Work out the finished part from the listing and answer in its coordinate system (mm). Face numbers are marked on the shaded views. Coordinates: 2 decimals unless noted, no trailing zeros. Order: outer loops, then holes, each group sorted by start corner. A loop starts at its lowest first (then second) coordinate and runs counter-clockwise, first axis right, second up. Notation, with made-up numbers: M 82,54.25 L 138,54.25 A27 ccw 138,73.25 Z; hole C 86.5,-3.5 d7. An arc over 180 degrees is marked long. Use a Markdown table: item, result.
from build123d import *

# Parameters (mm, degrees)
BOSS_EXTRUDE1_DEPTH = 55
SKETCH2_R           = 1.5
CUT_EXTRUDE1_DEPTH  = 10


with BuildPart() as part:
    # Sketch1 → Boss-Extrude1 (new body)
    with BuildSketch(Plane(origin=(0, 0, 0), x_dir=(1, 0, 0), z_dir=(0, 1, 0))):
        Polygon((3.175426481, 0), (1.58771324, 2.75), (-1.58771324, 2.75), (-3.175426481, 0), (-1.58771324, -2.75), (1.58771324, -2.75), align=None)
    extrude(amount=BOSS_EXTRUDE1_DEPTH)

    # Sketch2 → Cut-Extrude1 (cut)
    with BuildSketch(Plane(origin=(0, 55, 0), x_dir=(1, 0, 0), z_dir=(0, 1, 0))):
        with Locations(Location((0, 0, 0), (0, 0, 270))):
            Circle(SKETCH2_R)
    cut_extrude1 = extrude(amount=-CUT_EXTRUDE1_DEPTH, mode=Mode.SUBTRACT)

    # Mirror1: Cut-Extrude1 across plane
    add(cut_extrude1.mirror(Plane(origin=(0, 27.5, 0), x_dir=(0, 0, 1), z_dir=(0, -1, 0))), mode=Mode.SUBTRACT)


solid = part.part
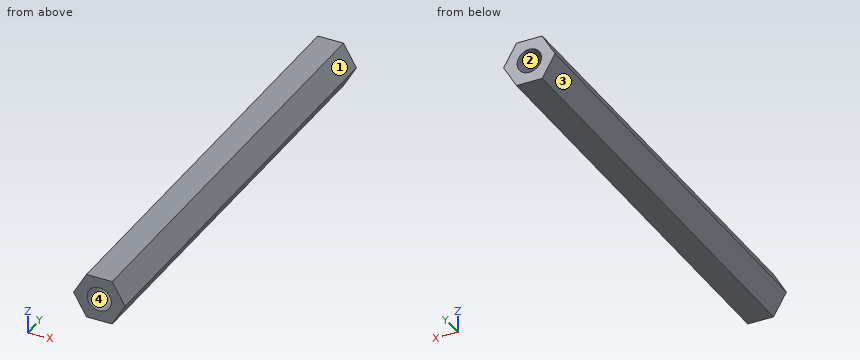
1. Section B-B on x = 0 is taken. Determine the outline of the cut face in (y, z).
Answers below:
| item | result |
|---|---|
| outline | M 0,-2.75 L 55,-2.75 L 55,-1.5 L 45,-1.5 L 45,1.5 L 55,1.5 L 55,2.75 L 0,2.75 L 0,1.5 L 10,1.5 L 10,-1.5 L 0,-1.5 Z |
2. Section C-C on y = 24.5 is taken. Determine the outline of the cut face in (x, z).
Answers below:
| item | result |
|---|---|
| outline | M -3.18,0 L -1.59,-2.75 L 1.59,-2.75 L 3.18,0 L 1.59,2.75 L -1.59,2.75 Z |
3. Section D-D on x = 2.25 is taken. Determine the outline of the cut face in (y, z), then the cut area to 3 significant figures.
Answers below:
| item | result |
|---|---|
| outline | M 0,-1.6 L 55,-1.6 L 55,1.6 L 0,1.6 Z |
| area | 176 mm² |
4. For a pull along X with two mould halves and no side action, classify the marked faces 1, 2, 3 and 4 as +X half, -X half, draft (parallel to the pull), parting line (faces both ways), or undercut.
Answers below:
| item | result |
|---|---|
| face 1 | +X half |
| face 2 | undercut |
| face 3 | -X half |
| face 4 | undercut |
5. Find the intervals of material crossed by probe 1 along X at (y, z) = (50.25, 0); probe 2 along Y at (x, z) = (0.25, 0.55); probe 3 along Z at (x, y) = (1, 9), in increasing order.
Answers below:
| item | result |
|---|---|
| probe 1 | -3.18 to -1.5, 1.5 to 3.18 |
| probe 2 | 10 to 45 |
| probe 3 | -2.75 to -1.12, 1.12 to 2.75 |
6. A flat-ended cylindrical pin translates along its axis: P1, Ø1.5, axis at x = 0, z = 0, coming from the -Y side. Find the tip coordinate at first contact, or state that the pin passes through.
Answers below:
| item | result |
|---|---|
| P1 | y = 10 |
7. Section A-A on y = 7.5 is taken. Determine the outline of the cut face in (x, z), then the cut area to 3 significant figures.
Answers below:
| item | result |
|---|---|
| outline | M -3.18,0 L -1.59,-2.75 L 1.59,-2.75 L 3.18,0 L 1.59,2.75 L -1.59,2.75 Z; hole C 0,0 d3 |
| area | 19.1 mm² |
